The listing builds one solid part. Answer for the finished solid, in the listing's coordinates (mm). A direction names the side the tool comes from. Round coordinates to 2 decimals unless told otherwise and drop trailing zeros. Order: outer loops, then holes, each group sorted by start corner. A loop starts at its lowest first (then second) coordinate and runs counter-clockwise, first axis right, second up. Notation, with made-up numbers: (-25, 22) -> (23, 22) arc R21 ccw to (23, 53) -> close; hole circle Ø4 at (40, 10.5). An arc over 180 degrees is marked (long way). Answer in a Markdown table with one row per item. Add a question column.
```python
from build123d import *

# Parameters (mm, degrees)
SKETCH1_W           = 70
SKETCH1_H           = 70
SKETCH1_R           = 4.6
SKETCH1_R_2         = 2
SKETCH1_R_3         = 4
BOSS_EXTRUDE1_DEPTH = 5
FILLET1_R           = 2
FILLET2_R           = 2
SKETCH2_R           = 5.85
CUT_EXTRUDE1_DEPTH  = 2.5


with BuildPart() as part:
    # Sketch1 → Boss-Extrude1 (new body)
    with BuildSketch(Plane.XY):
        Rectangle(SKETCH1_W, SKETCH1_H)
        Circle(SKETCH1_R, mode=Mode.SUBTRACT)
        with Locations((0, 27)):
            Circle(SKETCH1_R_2, mode=Mode.SUBTRACT)
        with Locations((0, -27)):
            Circle(SKETCH1_R_2, mode=Mode.SUBTRACT)
        with Locations((-27, 27)):
            Circle(SKETCH1_R_3, mode=Mode.SUBTRACT)
        with Locations((27, 27)):
            Circle(SKETCH1_R_3, mode=Mode.SUBTRACT)
        with Locations((27, -27)):
            Circle(SKETCH1_R_3, mode=Mode.SUBTRACT)
        with Locations((-27, -27)):
            Circle(SKETCH1_R_3, mode=Mode.SUBTRACT)
    extrude(amount=BOSS_EXTRUDE1_DEPTH)

    # Fillet1
    fillet1_edges = [part.edges().sort_by_distance(p)[0] for p in [
        (-35, 35, 2.5),
        (35, 35, 2.5),
        (35, -35, 2.5),
    ]]
    fillet(fillet1_edges, radius=FILLET1_R)

    # Fillet2
    fillet2_edges = [part.edges().sort_by_distance(p)[0] for p in [
        (-35, -35, 2.5),
    ]]
    fillet(fillet2_edges, radius=FILLET2_R)

    # Sketch2 → Cut-Extrude1 (cut)
    with BuildSketch(Plane.XY.offset(5)):
        with Locations((-27, 27)):
            Circle(SKETCH2_R)
        with Locations((27, 27)):
            Circle(SKETCH2_R)
        with Locations((27, -27)):
            Circle(SKETCH2_R)
        with Locations((-27, -27)):
            Circle(SKETCH2_R)
    extrude(amount=-CUT_EXTRUDE1_DEPTH, mode=Mode.SUBTRACT)


solid = part.part
```
1. Straight lines are drawn through the part: line 1 along Y through (x, z) = (-27, 1.15); line 2 along Y through (x, z) = (27, 3.35); line 3 along X through (y, z) = (-31, 3.15). For each, find the intervals that lie inside material, in ascending order.
2. Each of these flat-tipped pins is pushed along its axis until it touches: pin 1 (9.5 mm diameter, centred on x = -28.5, y = -27, fed in from +Z); pin 2 (3.5 mm diameter, centred on x = 26.5, y = -29.5, fed in from +Z). Where does it stop, or does it pass through?
3. For faces 1 (the cylindrical face through (-23.855, 31.933, 3.768)), 2 (the cylindrical face through (24.05, 29.7, 1.23)), determine the directions among +Z, -Z, +X, -X, +Y, -Y from which every point of the face is accessible in a straight line to the end or side of a thin tool.
4. The part is cut by section A-A (x = -27). Give the vertices of the cut face in (y, z).
5. The mould has two halves that part along X. Classify faces 3 (the flat face through (0, -35, 2)), 4 (the cylindrical face through (26.24, 32.8, 3.77)), 5 (the cylindrical face through (-34.43, 34.4, 2.54)): released by +X, released by -X, zero draft, split by the parting line, or undercut.
6. The part is cut by section C-C (z = 4). Give the vertices of the cut face in (x, y), then the cut area to 3 significant figures.
7. The part is cut by section B-B (y = 27). Give the vertices of the cut face in (x, z).
Report:
| question | item | result |
|---|---|---|
| 1 | line 1 | y = -35 to -31, -23 to 23, 31 to 35 |
| 1 | line 2 | y = -35 to -32.85, -21.15 to 21.15, 32.85 to 35 |
| 1 | line 3 | x = -35 to -31.27, -22.73 to 22.73, 31.27 to 35 |
| 2 | pin 1 | stops at z = 5 |
| 2 | pin 2 | stops at z = 2.5 |
| 3 | face 1 | +Z |
| 3 | face 2 | +Z, -Z |
| 4 | outline | (-35, 0) -> (-31, 0) -> (-31, 2.5) -> (-32.85, 2.5) -> (-32.85, 5) -> (-35, 5) -> close; (-23, 0) -> (23, 0) -> (23, 2.5) -> (21.15, 2.5) -> (21.15, 5) -> (-21.15, 5) -> (-21.15, 2.5) -> (-23, 2.5) -> close; (31, 0) -> (35, 0) -> (35, 5) -> (32.85, 5) -> (32.85, 2.5) -> (31, 2.5) -> close |
| 5 | face 3 | zero draft |
| 5 | face 4 | undercut |
| 5 | face 5 | released by -X |
| 6 | outline | (-35, -33) arc R2 ccw to (-33, -35) -> (33, -35) arc R2 ccw to (35, -33) -> (35, 33) arc R2 ccw to (33, 35) -> (-33, 35) arc R2 ccw to (-35, 33) -> close; hole circle Ø11.7 at (-27, -27); hole circle Ø11.7 at (-27, 27); hole circle Ø9.2 at (0, 0); hole circle Ø4 at (0, -27); hole circle Ø4 at (0, 27); hole circle Ø11.7 at (27, -27); hole circle Ø11.7 at (27, 27) |
| 6 | area | 4,370 mm^2 |
| 7 | outline | (-35, 0) -> (-31, 0) -> (-31, 2.5) -> (-32.85, 2.5) -> (-32.85, 5) -> (-35, 5) -> close; (-23, 0) -> (-2, 0) -> (-2, 5) -> (-21.15, 5) -> (-21.15, 2.5) -> (-23, 2.5) -> close; (2, 0) -> (23, 0) -> (23, 2.5) -> (21.15, 2.5) -> (21.15, 5) -> (2, 5) -> close; (31, 0) -> (35, 0) -> (35, 5) -> (32.85, 5) -> (32.85, 2.5) -> (31, 2.5) -> close |
